Input: dimensioned drawing with shaded views. Units: mm. Origin: part minimum x, y, z. Round coordinates to 2 decimals unless told otherwise and drop trailing zeros. Write each loop counter-clockwise with the first axis right and the second up, starting at its lowest first coordinate (ties: lowest second). Pieces come first, ordered by that corner, then holes. Notation, with made-up numbers: (47, 59) -> (97, 59) arc R30 cw to (97, 89) -> close; hole circle Ø9 at (16.25, -2). An arc over 180 degrees is marked (long way). Return JSON: item names as keys, results as strings. Group by question number.
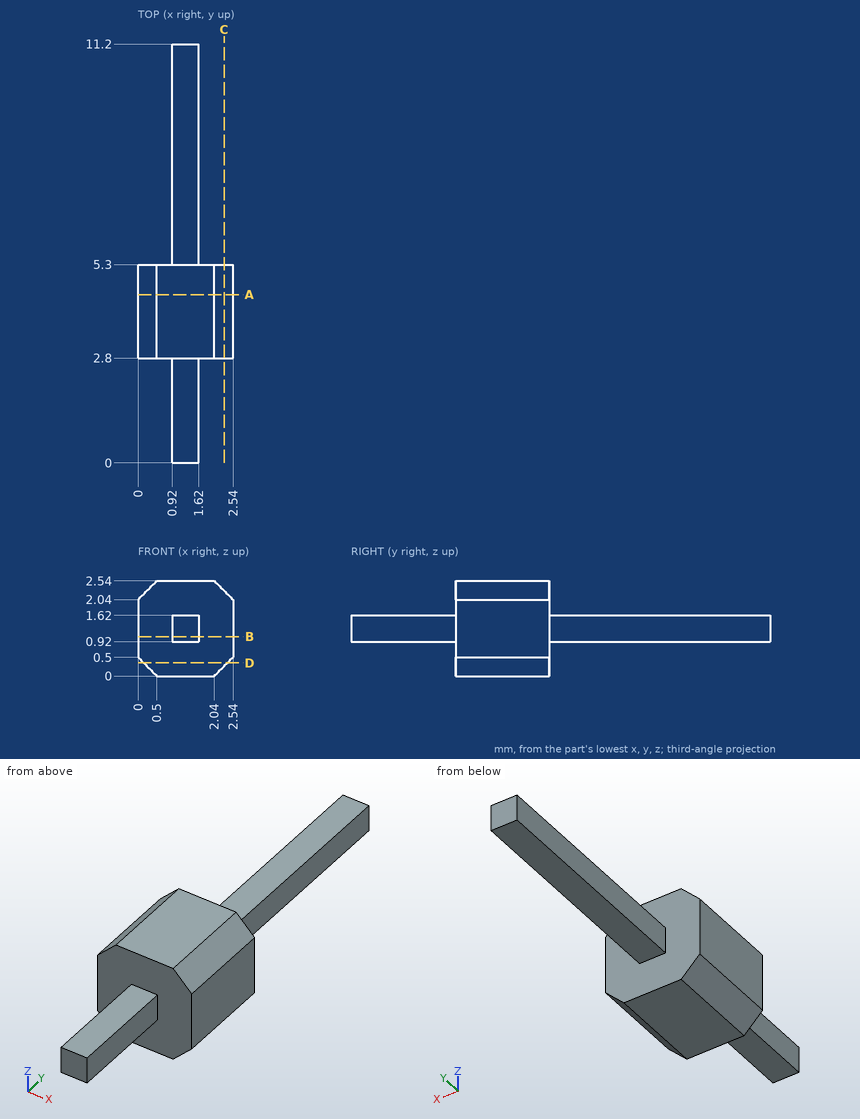
Item 1: Cut plane A-A on y = 4.5. Output: boundary loops of the cut face in (x, z), and give its area (3 significant figures).
Item 2: Cut plane C-C on x = 2.3. Output: boundary loops of the cut face in (y, z), and give its area (3 significant figures).
Item 3: Cut plane B-B on z = 1.05. Output: boundary loops of the cut face in (x, y), and give its area (3 significant figures).
Item 4: First-contact query: pin 1 Ø0.6 at (x, y) = (1, 2) entering from -Z; pin 2 Ø0.8 at (x, y) = (1.5, 1) entering from +Z; pin 3 Ø1 at (x, y) = (1.5, 4) entering from -Z; pin 4 Ø0.6 at (y, z) = (8, 1.5) entering from -X. Flat tips, straight axial feed; report the tip coordinate or a pass-through.
Item 5: Material intervals for probe 1 along Z at (x, y) = (1.2, 6.25); probe 2 along Y at (x, z) = (2.15, 0.7), sorted ascending.
Item 6: Cut plane D-D on z = 0.35. Output: boundary loops of the cut face in (x, y), and give its area (3 significant figures).
Here are the results:
{
 "1": {"outline": "(0, 0.5) -> (0.5, 0) -> (2.04, 0) -> (2.54, 0.5) -> (2.54, 2.04) -> (2.04, 2.54) -> (0.5, 2.54) -> (0, 2.04) -> close", "area": "5.95 mm^2"},
 "2": {"outline": "(2.8, 0.26) -> (5.3, 0.26) -> (5.3, 2.28) -> (2.8, 2.28) -> close", "area": "5.05 mm^2"},
 "3": {"outline": "(0, 2.8) -> (0.92, 2.8) -> (0.92, 0) -> (1.62, 0) -> (1.62, 2.8) -> (2.54, 2.8) -> (2.54, 5.3) -> (1.62, 5.3) -> (1.62, 11.2) -> (0.92, 11.2) -> (0.92, 5.3) -> (0, 5.3) -> close", "area": "12.4 mm^2"},
 "4": {"pin 1": "stops at z = 0.92", "pin 2": "stops at z = 1.62", "pin 3": "stops at z = 0", "pin 4": "stops at x = 0.92"},
 "5": {"probe 1": "z = 0.92 to 1.62", "probe 2": "y = 2.8 to 5.3"},
 "6": {"outline": "(0.15, 2.8) -> (2.39, 2.8) -> (2.39, 5.3) -> (0.15, 5.3) -> close", "area": "5.60 mm^2"}
}
